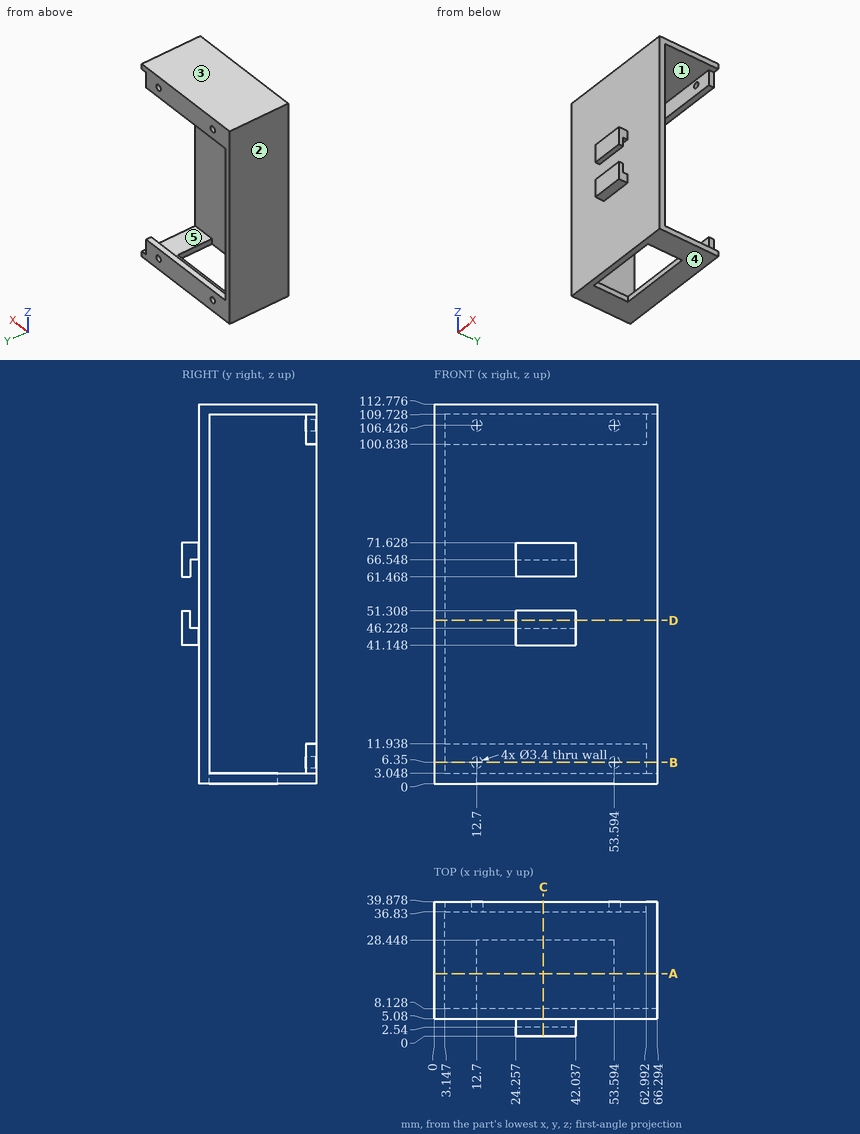
Here's the drawing with two shaded views (mm, measured from the low corner). I have some questions. A direction names the side the tool comes from. Round coordinates to 2 decimals unless told otherwise and drop trailing zeros. Loops run counter-clockwise (first coordinate to the right, second up) from the corner with the lowest first, then second, coordinate; pieces in that order, holes last. Notation, with made-up numbers: (-6, 70.5) - (26, 70.5) arc R33 ccw to (26, 99.5) - close; hole circle Ø10 at (-9, -24). An arc over 180 degrees is marked (long way). Write item = value, one per line.
1) Imagine slicing it at D-D (z = 48.5). Please give me the cut outline in (x, y), and give its area (3 significant figures).
Computed:
outline = (0, 5.08) - (66.29, 5.08) - (66.29, 8.13) - (3.15, 8.13) - (3.15, 39.88) - (0, 39.88) - close; (24.26, 0) - (42.04, 0) - (42.04, 2.54) - (24.26, 2.54) - close
area = 347 mm2
2) I need wall thicknesses on line 1 along Z through (x, y) = (12.7, 39.05); line 2 along X through (y, z) = (38.3, 6.35); line 3 along Z through (x, y) = (6, 33.5). Which ranges of each line are inside material? Lowest first, please. Write a range as from..to.
Computed:
line_1 = 0..4.65, 8.05..11.94, 100.84..104.73, 108.13..112.78
line_2 = 0..11, 14.4..51.89, 55.29..62.99
line_3 = 0..3.05, 109.73..112.78
3) If we mould it in two halves opening along Z, with no side actions, what happens to the marked faces 3, 4 and 5? For each: pulls with the +Z half, pulls with the -Z half, needs draft (parallel to the pull), parting line crosses it, or undercut.
Computed:
face_3 = pulls with the +Z half
face_4 = pulls with the -Z half
face_5 = undercut
4) Imagine slicing it at A-A (y = 18.5). Please give me the cut outline in (x, z), and give its area (3 significant figures).
Computed:
outline = (0, 0) - (12.7, 0) - (12.7, 3.05) - (3.15, 3.05) - (3.15, 109.73) - (66.29, 109.73) - (66.29, 112.78) - (0, 112.78) - close; (53.59, 0) - (66.29, 0) - (66.29, 3.05) - (53.59, 3.05) - close
area = 615 mm2
5) Imagine slicing it at B-B (z = 6.35). Please give me the cut outline in (x, y), and give its area (3 significant figures).
Computed:
outline = (0, 5.08) - (66.29, 5.08) - (66.29, 8.13) - (3.15, 8.13) - (3.15, 36.83) - (11, 36.83) - (11, 39.88) - (0, 39.88) - close; (14.4, 36.83) - (51.89, 36.83) - (51.89, 39.88) - (14.4, 39.88) - close; (55.29, 36.83) - (62.99, 36.83) - (62.99, 39.88) - (55.29, 39.88) - close
area = 464 mm2
6) On a 3-axis mill with a long thin cutter (end or side, diameter ignored), from which of +Z, -Z, +X, -X, +Y, -Y can I reach the whole of each face in a straight line? I mean the marked faces 1 and 2. Say none if no direction works.
Computed:
face_1 = +X
face_2 = +Z, -Z, -X, +Y, -Y
7) Imagine slicing it at C-C (x = 32.5). Please give me the cut outline in (y, z).
Computed:
outline = (0, 41.15) - (5.08, 41.15) - (5.08, 0) - (8.13, 0) - (8.13, 109.73) - (36.83, 109.73) - (36.83, 100.84) - (39.88, 100.84) - (39.88, 112.78) - (5.08, 112.78) - (5.08, 71.63) - (0, 71.63) - (0, 61.47) - (2.54, 61.47) - (2.54, 66.55) - (5.08, 66.55) - (5.08, 46.23) - (2.54, 46.23) - (2.54, 51.31) - (0, 51.31) - close; (28.45, 0) - (39.88, 0) - (39.88, 11.94) - (36.83, 11.94) - (36.83, 3.05) - (28.45, 3.05) - close
8) I'm going to push flat-ended pins straight in: P1, Ø3.5, axis at y = 38, z = 8.5, coming from the +X side; P2, Ø1, axis at x = 39.5, z = 95.5, coming from the -Y side; P3, Ø1.5, axis at x = 33, y = 4, coming from the +Z side. Where does each tip first touch, or does it pass through?
Computed:
P1 = 62.99
P2 = 5.08
P3 = 71.63
